Autodesk Inventor part; units mm, degrees
ref_plane "YZ Plane" through (0, 0, 0) normal (1, 0, 0) x (0, 1, 0)
ref_plane "XZ Plane" through (0, 0, 0) normal (0, 1, 0) x (-1, 0, 0)
ref_plane "XY Plane" through (0, 0, 0) normal (0, 0, 1) x (1, 0, 0)
sketch "Sketch1" plane through (0, 0, 0) normal (1, 0, 0) x (0, 1, 0)
  arc A0 (-28, 0) -> (28, 0) centre (0, 0) ccw
  line L0 (-28, 0) -> (28, 0) construction
  line L1 (28, 0) -> (28, 96)
  line L2 (28, 96) -> (-28, 96)
  line L3 (-28, 96) -> (-28, 0)
  circle A1 centre (0, 0) radius 7.05
  circle A2 centre (8, 8) radius 2.1
  circle A3 centre (-8, 8) radius 2.1
  circle A4 centre (-8, -8) radius 2.1
  circle A5 centre (8, -8) radius 2.1
  circle A6 centre (12, 92) radius 2.1
  line L4 (0, 96) -> (0, 0) construction
  circle A7 centre (-20, 92) radius 2
  dimension "d0" = 28
  dimension "d1" = 96
  dimension "d2" = 14.1
  dimension "d3" = 4.2
  dimension "d4" = 8
  dimension "d5" = 8
  dimension "d8" = 360
  dimension "d10" = 4.2
  dimension "d11" = 12
  dimension "d12" = 4
  dimension "d43" = 4
  dimension "d44" = 32
extrude "Extrusion1" add sketch "Sketch1" along normal blind 3
sketch "Sketch2" plane through (3, 0, 0) normal (1, 0, 0) x (0, 0, -1)
  line L0 (-76.9, 35.5) -> (-76.9, -13) construction
  line L1 (-76.9, -13) -> (-76.9, 0) construction
  line L2 (-79.4, 35.25) -> (-74.4, 35.25) construction
  line L3 (-74.4, 35.25) -> (-74.4, -12.75) construction
  line L4 (-74.4, -12.75) -> (-79.4, -12.75) construction
  line L5 (-79.4, -12.75) -> (-79.4, 35.25) construction
  line L6 (-79.4, 35.25) -> (-74.4, -12.75) construction
  line L7 (-74.4, 35.25) -> (-79.4, -12.75) construction
  line L8 (0, 28) -> (-96, 28)
  line L9 (-96, 28) -> (-96, 40)
  line L10 (-96, 40) -> (0, 40)
  line L11 (0, 40) -> (0, 28)
  circle A0 centre (-76.9, 35.25) radius 2.1
  circle A1 centre (-76.9, -12.75) radius 2.1
  circle A2 centre (-92, 12) radius 2.1
  point P0 (0, 0)
  point P1 (-76.9, 11.25)
  dimension "d17" = 48.5
  dimension "d18" = 13
  dimension "d19" = 5
  dimension "d20" = 48
  dimension "d22" = 12
  dimension "d24" = 4.2
  dimension "d31" = 4.2
  dimension "d34" = 15.1
extrude "Extrusion2" add sketch "Sketch2" against normal up to surface (3 mm away) contours L8 L9 L10 L11
fillet "Fillet1" radius 6 1 edges at (1.5, 28, 0)
fillet "Fillet2" radius 6 1 edges at (1.5, 40, 0)
extrude "Extrusion4" cut sketch "Sketch2" against normal through all contours A1
sketch "Sketch3" plane through (3, 0, 0) normal (1, 0, 0) x (0, 0, -1)
  line L0 (-96, -28) -> (-96, 40)
  line L1 (-6, 40) -> (-96, 40)
  line L2 (-96, 24) -> (-84, 24)
  line L3 (-84, 24) -> (-84, 40)
  point P0 (0, 0)
  dimension "d37" = 12
  dimension "d38" = 16
extrude "Extrusion5" cut sketch "Sketch3" against normal through all
fillet "Fillet3" radius 8 2 edges at (1.5, 24, 84) (1.5, 40, 84)
fillet "Fillet4" radius 6 1 edges at (1.5, 24, 96)
properties part number "EndEffectorStage1Plate" material "Aluminum 6061"
For this review, take the finished solid that the model builds, in its own axes (mm). Coordinates: 2 decimals unless noted, no trailing zeros. Loops run counter-clockwise (first coordinate to the right, second up) from the corner with the lowest first, then second, coordinate; pieces in that order, holes last. Notation, with made-up numbers: (-33, 58) -> (0, 58) arc R21 ccw to (0, 86) -> close; hole circle Ø8 at (24, 11.25). An arc over 180 degrees is marked (long way). Return JSON: item names as keys, results as strings. Group by question number.
(1) To check wall thickness, follow L1, parallel to Z at x = 2.2, y = 0; L2, parallel to Y at x = 2, z = 76.9; L3, parallel to Z at x = 1.2, y = 8. State the ranges of each line that lie inside material, in increasing order.
(2) Consider section A-A, the plane y = 0. Give the boundary of the cut face in (x, z).
(3) Consider section D-D, the plane z = -16.5. Give the boundary of the cut face in (x, y), plus the area to 3 significant figures.
(4) Consider section B-B, the plane y = -12.75. Give the boundary of the cut face in (x, z), plus the area to 3 significant figures.
(5) Mouldability with a two-part tool opening along Z and no side actions: class faces 1 (the flat face through (0, 6, 35)), 2 (the cylindrical face through (1.479, 7.727, 5.918)), 3 (the cylindrical face through (1.52, 29.66, -1.36)) as pulls with the +Z half, pulls with the -Z half, needs draft (parallel to the pull), parting line crosses it, or undercut.
(6) Consider section C-C, the plane x = 1.05. Count the separate pieces of the cut face and the enclosed holes in it, plus the area to 3 significant figures.
(7) For pin 1 Ø5.5 at (y, z) = (-8, 8) entering from -X; pin 2 Ø4 at (y, z) = (8, 8) entering from +X, all flat-tipped, find the tip position at first contact; note any pin that passes through.
Results below:
{
 "1": {"L1": "z = -28 to -7.05, 7.05 to 96", "L2": "y = -28 to -14.85, -10.65 to 33.15, 37.35 to 39.95", "L3": "z = -26.83 to -10.1, -5.9 to 5.9, 10.1 to 96"},
 "2": {"outline": "(0, -28) -> (3, -28) -> (3, -7.05) -> (0, -7.05) -> close; (0, 7.05) -> (3, 7.05) -> (3, 96) -> (0, 96) -> close"},
 "3": {"outline": "(0, -22.62) -> (3, -22.62) -> (3, 22.62) -> (0, 22.62) -> close", "area": "136 mm2"},
 "4": {"outline": "(0, -24.93) -> (3, -24.93) -> (3, 74.8) -> (0, 74.8) -> close; (0, 79) -> (3, 79) -> (3, 96) -> (0, 96) -> close", "area": "350 mm2"},
 "5": {"face 1": "needs draft", "face 2": "undercut", "face 3": "pulls with the -Z half"},
 "6": {"separate pieces": "1", "enclosed holes": "9", "area": "7,290 mm2"},
 "7": {"pin 1": "stops at x = 0", "pin 2": "passes through"}
}
